Model file for the job. Use its own axes, mm. Face numbers are marked on the shaded views. Coordinates: 2 decimals unless noted, no trailing zeros. Write each loop counter-clockwise with the first axis right and the second up, starting at its lowest first coordinate (ties: lowest second). Pieces come first, ordered by that corner, then holes. Notation, with made-up numbers: M -1,-19 L 23,-19 A28 cw 23,8 Z; hole C -20,54.25 d5. An arc over 180 degrees is marked long. Put each result on its own line as item: value. Start each with the question number.
Q1. Cut at A-A (z = 0). Write the cut outline in (x, y), then the cut area to 4 significant figures.
Q2. Cut at C-C (y = 3). Write the cut outline in (x, z), then the cut area to 3 significant figures.
Q3. Pull direction X, two halves, no side cores. Call the marked faces 1, 2 and 3: pulls with the +X half, pulls with the -X half, needs draft (parallel to the pull), parting line crosses it, or undercut.
Q4. Drill centre lines: line 1 along Y through (x, z) = (0.7, -0.4); line 2 along Y through (x, z) = (-0.8, -1.15); line 3 along Y through (x, z) = (1, -1.9). Where is each one in solid material? Low to high.
Q5. Cut at B-B (x = 0). Write the cut outline in (y, z).
Q6. Drop flat-ended pins along their axis: pin 1 (3 mm diameter, centred on y = 10.5, z = -2, fed in from -X); pin 2 (1.2 mm diameter, centred on x = -0.5, y = 19.5, fed in from -Z); pin 3 (1.2 mm diameter, centred on x = 0.5, y = 19.5, fed in from +Z); pin 4 (3 mm diameter, centred on x = 0, z = 0, fed in from +Y). Give the stop position or say it passes through.
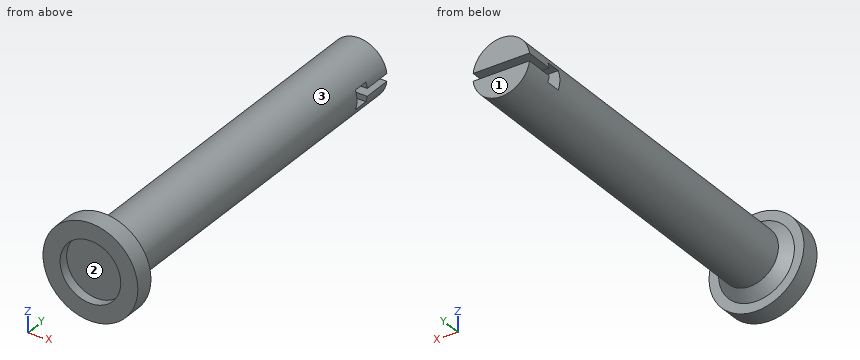
Autodesk Inventor part; units mm, degrees
ref_plane "YZ Plane" through (0, 0, 0) normal (1, 0, 0) x (0, 1, 0)
ref_plane "XZ Plane" through (0, 0, 0) normal (0, 1, 0) x (-1, 0, 0)
ref_plane "XY Plane" through (0, 0, 0) normal (0, 0, 1) x (1, 0, 0)
sketch "Sketch1" plane through (0, 0, 0) normal (0, 0, 1) x (1, 0, 0)
  line L0 (0, 0) -> (0, 26)
  line L1 (0, 26) -> (1.5, 26)
  line L2 (1.5, 26) -> (1.5, 1)
  line L3 (1.5, 1) -> (2.5, 1)
  line L4 (2.5, 1) -> (2.5, 0)
  line L5 (2.5, 0) -> (0, 0)
  line L6 (1.5, 26) -> (4, 26)
  line L7 (4, 26) -> (4, 24)
  line L8 (4, 24) -> (1.5, 24)
  line L9 (1.5, 24) -> (1.5, 26)
  point P0 (1.5, 24)
  dimension "d0" = 2.5
  dimension "d1" = 1.5
  dimension "d2" = 1
  dimension "d3" = 26
  dimension "d5" = 2
  dimension "d6" = 4
revolve "Revolution1" add sketch "Sketch1" angle 360 about axis through (0, 0, 0) along (0, 1, 0) contours L0 L1 L2 L3 L4 L5
sketch "Sketch2" plane through (0, 0, 0) normal (0, -1, 0) x (1, 0, 0)
  circle A0 centre (0, 0) radius 1.6
  dimension "d10" = 3.2
extrude "Extrusion1" cut sketch "Sketch2" against normal blind 0.5
chamfer "Chamfer1" distance 0.5 angle 45 1 edges at (-1.5, 1, 0)
sketch "Sketch3" plane through (0, 0, 0) normal (1, 0, 0) x (0, 1, 0)
  line L0 (1.5, 1.5) -> (26, 1.5)
  line L1 (20.5, 1.5) -> (20.5, 0.2)
  line L2 (20.5, 0.2) -> (19, 0.2)
  line L3 (19, 0.2) -> (19, 0.5)
  line L4 (19, 0.5) -> (18.2, 0.5)
  line L5 (18.2, 0.5) -> (18.2, -0.5)
  line L6 (18.2, -0.5) -> (19, -0.5)
  line L7 (19, -0.5) -> (19, -0.2)
  line L8 (19, -0.2) -> (20.5, -0.2)
  line L9 (20.5, -0.2) -> (20.5, -1.5)
  line L10 (1.5, -1.5) -> (26, -1.5)
  line L11 (26, 0) -> (62.914, 0) construction
  line L12 (20.5, 1.5) -> (26, 1.5)
  line L13 (1.5, 1.5) -> (26, 1.5)
  line L14 (26, -1.5) -> (26, 1.5)
  line L15 (26, -1.5) -> (26, 1.5)
  line L16 (26, 1.5) -> (26, -1.5)
  line L17 (20.5, -1.5) -> (26, -1.5)
  line L18 (26, 0) -> (18.2, 0) construction
  point P0 (0, 0)
  dimension "d16" = 0.4
  dimension "d17" = 1.5
  dimension "d18" = 0.8
  dimension "d19" = 1
  dimension "d23" = 5.5
  dimension "d24" = 1.3
extrude "Extrusion2" cut sketch "Sketch3" along normal mid plane 10
properties part number "Taster"
Computed values:
1. outline: M -2.5,0 L -1.6,0 L -1.6,0.5 L 1.6,0.5 L 1.6,0 L 2.5,0 L 2.5,1 L 2,1 L 1.5,1.5 L 1.5,18.2 L -1.5,18.2 L -1.5,1.5 L -2,1 L -2.5,1 Z
1. area: 55.25 mm2
2. outline: C 0,0 d3
2. area: 7.07 mm2
3. face 1: needs draft
3. face 2: undercut
3. face 3: parting line crosses it
4. line 1: 0.5 to 18.2, 19 to 20.5
4. line 2: 0.5 to 20.5
4. line 3: 0 to 1
5. outline: M 0,-2.5 L 1,-2.5 L 1,-2 L 1.5,-1.5 L 20.5,-1.5 L 20.5,-0.2 L 19,-0.2 L 19,-0.5 L 18.2,-0.5 L 18.2,0.5 L 19,0.5 L 19,0.2 L 20.5,0.2 L 20.5,1.5 L 1.5,1.5 L 1,2 L 1,2.5 L 0,2.5 L 0,1.6 L 0.5,1.6 L 0.5,-1.6 L 0,-1.6 Z
6. pin 1: x = -1.41
6. pin 2: z = -1.5
6. pin 3: z = 1.5
6. pin 4: y = 20.5
